The listing builds one solid part. Answer for the finished solid, in the listing's coordinates (mm). Round coordinates to 2 decimals unless told otherwise and drop trailing zeros. Write each loop counter-clockwise with the first axis right and the second up, starting at its lowest first coordinate (ties: lowest second). Pieces come first, ordered by that corner, then holes.
Item 1: Find the intervals of material crossed by probe 1 along X at (y, z) = (1.35, 18); probe 2 along X at (y, z) = (4.3, 19), in increasing order.
Item 2: Find section D-D on x = -19. Give the vertices of the cut face in (y, z), then the cut area to 3 significant figures.
Item 3: Find section A-A on y = 0.8. Give the vertices of the cut face in (x, z), then the cut area to 3 significant figures.
Item 4: Find section B-B on z = 0. Give the vertices of the cut face in (x, y).
Item 5: Each of these flat-tipped pins is pushed along its axis until it touches: pin 1 (3 mm diameter, centred on x = 22.5, z = -22.5, fed in from +Y); pin 2 (4 mm diameter, centred on x = 19, z = 19, fed in from +Y); pin 3 (1 mm diameter, centred on x = -3.5, y = 3, fed in from +Z). Where does it stop, or does it pass through?
Item 6: For a pull along X with two mould halves and no side action, classify faces 1 (the face through (-4.036, 2.465, 30.736)), 2 (the face through (-3.855, 2.535, 0.226)), 3 (the face through (19.47, 3.68, -21.1)), 4 (the face through (0, 0, 0)) as +X half, -X half, draft (parallel to the pull), parting line (faces both ways), or undercut.
Item 7: Find section C-C on x = 8. Give the vertices of the cut face in (y, z), then the cut area to 3 significant figures.
```python
from build123d import *

# Parameters (mm, degrees)
F0_R           = 31
F1_DEPTH       = 5
F2_D           = 10.3
F3_D           = 4.3
F3_CSINK_D     = 8.96
F3_CSINK_ANGLE = 90


with BuildPart() as f1:
    # F0 (on Front) → F1 (new body)
    with BuildSketch(Plane.XZ):
        Circle(F0_R)
    extrude(amount=-F1_DEPTH)

    # F2 (through all)
    with Locations(Plane.XZ):
        with Locations((-9, 0), (9, 0)):
            Hole(F2_D / 2)

    # F3 (through all)
    with Locations(Plane.XZ):
        with Locations((-19, 19), (19, 19), (19, -19), (-19, -19)):
            CounterSinkHole(F3_D / 2, F3_CSINK_D / 2, counter_sink_angle=F3_CSINK_ANGLE)


solid = f1.part
```
Check values:
1. probe 1: x = -25.24 to -21.97, -16.03 to 16.03, 21.97 to 25.24
1. probe 2: x = -24.49 to -21.15, -16.85 to 16.85, 21.15 to 24.49
2. outline: (0, -24.49) - (5, -24.49) - (5, -21.15) - (2.33, -21.15) - (0, -23.48) - close; (0, -14.52) - (2.33, -16.85) - (5, -16.85) - (5, 16.85) - (2.33, 16.85) - (0, 14.52) - close; (0, 23.48) - (2.33, 21.15) - (5, 21.15) - (5, 24.49) - (0, 24.49) - close
2. area: 191 mm2
3. outline: circle Ø62 at (0, 0); hole circle Ø7.36 at (-19, -19); hole circle Ø7.36 at (-19, 19); hole circle Ø10.3 at (-9, 0); hole circle Ø10.3 at (9, 0); hole circle Ø7.36 at (19, -19); hole circle Ø7.36 at (19, 19)
3. area: 2,680 mm2
4. outline: (-31, 0) - (-14.15, 0) - (-14.15, 5) - (-31, 5) - close; (-3.85, 0) - (3.85, 0) - (3.85, 5) - (-3.85, 5) - close; (14.15, 0) - (31, 0) - (31, 5) - (14.15, 5) - close
5. pin 1: stops at y = 5
5. pin 2: passes through
5. pin 3: stops at z = 30.85
6. face 1: parting line
6. face 2: undercut
6. face 3: undercut
6. face 4: draft
7. outline: (0, -29.95) - (5, -29.95) - (5, -5.05) - (0, -5.05) - close; (0, 5.05) - (5, 5.05) - (5, 29.95) - (0, 29.95) - close
7. area: 249 mm2
